Geometry: final body of the model. Coordinates: model frame, mm. A direction names the side the tool comes from. Coordinates: 2 decimals unless noted, no trailing zeros. Write each loop counter-clockwise with the first axis right and the second up, starting at its lowest first coordinate (ties: lowest second). Pieces come first, ordered by that corner, then holes.
from build123d import *

# Parameters (mm, degrees)
EXTRUDE_THIN1_DEPTH = 2
SKETCH2_R           = 3
BOSS_EXTRUDE1_DEPTH = 2
SKETCH3_R           = 1.5
CUT_EXTRUDE1_DEPTH  = 23.73845331
SKETCH4_R           = 1.5
BOSS_EXTRUDE2_DEPTH = 2.1
EXTRUDE_THIN2_DEPTH = 2
EXTRUDE_THIN3_DEPTH = 2
SKETCH7_W           = 1.2
SKETCH7_H           = 23.975911633
EXTRUDE_THIN4_DEPTH = 2


with BuildPart() as part:
    # Sketch1 → Extrude-Thin1 (new body)
    with BuildSketch(Plane(origin=(0, 0, 0), x_dir=(1, 0, 0), z_dir=(0, 1, 0))):
        Polygon((-2.187026997, 14.752740827), (-17.187026997, -11.228021286), (12.812973003, -11.228021286), align=None)
        Polygon((-2.187026997, 12.352740827), (-15.108566028, -10.028021286), (10.734512034, -10.028021286), align=None, mode=Mode.SUBTRACT)
    extrude(amount=EXTRUDE_THIN1_DEPTH)

    # Sketch2 → Boss-Extrude1 (add)
    with BuildSketch(Plane(origin=(0, 0, 0), x_dir=(1, 0, 0), z_dir=(0, 1, 0))):
        with Locations((-9.687026997, 1.76235977)):
            Circle(SKETCH2_R)
        with Locations((5.312973003, 1.76235977)):
            Circle(SKETCH2_R)
        with Locations((-2.187026997, -11.228021286)):
            Circle(SKETCH2_R)
    extrude(amount=BOSS_EXTRUDE1_DEPTH)

    # Sketch3 → Cut-Extrude1 (cut, through all)
    with BuildSketch(Plane(origin=(0, 0, 0), x_dir=(1, 0, 0), z_dir=(0, 1, 0))):
        with Locations(Location((-9.687026997, 1.76235977, 0), (0, 0, 270))):
            Circle(SKETCH3_R)
        with Locations(Location((5.312973003, 1.76235977, 0), (0, 0, 270))):
            Circle(SKETCH3_R)
    extrude(amount=CUT_EXTRUDE1_DEPTH, mode=Mode.SUBTRACT)

    # Sketch4 → Boss-Extrude2 (add)
    with BuildSketch(Plane(origin=(0, 2, 0), x_dir=(1, 0, 0), z_dir=(0, 1, 0))):
        with Locations(Location((-2.187026997, -11.228021286, 0), (0, 0, 270))):
            Circle(SKETCH4_R)
    extrude(amount=BOSS_EXTRUDE2_DEPTH)

    # Sketch5 → Extrude-Thin2 (add)
    with BuildSketch(Plane(origin=(0, 0, 0), x_dir=(1, 0, 0), z_dir=(0, 1, 0))):
        Polygon((-5.388180626, 8.61177443), (2.926064281, 1.202897678), (-10.696610006, -3.999977956), (-6.443313294, -10.266536854), (-7.436211418, -10.940445836), (-12.540725216, -3.419753411), (0.654437519, 1.619843752), (-6.186526415, 7.715870417), align=None)
    extrude_thin2 = extrude(amount=EXTRUDE_THIN2_DEPTH)

    # Sketch6 → Extrude-Thin3 (add)
    with BuildSketch(Plane(origin=(0, 0, 0), x_dir=(1, 0, 0), z_dir=(0, 1, 0))):
        Polygon((-15.108566028, -10.028021286), (6.483160233, -1.838837543), (6.05761065, -0.716827048), (-15.534115611, -8.906010791), align=None)
    extrude_thin3 = extrude(amount=EXTRUDE_THIN3_DEPTH)

    # Mirror1: Extrude-Thin2, Extrude-Thin3 across plane
    add(extrude_thin2.mirror(Plane(origin=(-2.187026997, 0, 0), x_dir=(0, 0, 1), z_dir=(1, 0, 0))))
    add(extrude_thin3.mirror(Plane(origin=(-2.187026997, 0, 0), x_dir=(0, 0, 1), z_dir=(1, 0, 0))))

    # Sketch7 → Extrude-Thin4 (add)
    with BuildSketch(Plane(origin=(0, 0, 0), x_dir=(1, 0, 0), z_dir=(0, 1, 0))):
        with Locations((-2.187026997, 0.75993453)):
            Rectangle(SKETCH7_W, SKETCH7_H)
    extrude(amount=EXTRUDE_THIN4_DEPTH)


solid = part.part
Item 1: Set-up query: faces 1 (the flat face through (7, 1, 11.228)), 2 (the flat face through (-11, 1, 11.228)), 3 (the flat face through (-12, 1, 10.028)). Return all of +Z, -Z, +X, -X, +Y, -Y with unobstructed straight access to the full face (end or side cutting, diameter ignored); none if empty.
Derived:
face 1: +Z, +X, +Y, -Y
face 2: +Z, -X, +Y, -Y
face 3: +Y, -Y
Item 2: Section C-C, the plane z = 5. Output: boundary loops of the cut face in (x, y).
Derived:
outline: (-13.59, 0) - (-12.21, 0) - (-12.21, 2) - (-13.59, 2) - close; (-11.47, 0) - (-10.02, 0) - (-10.02, 2) - (-11.47, 2) - close; (-5.24, 0) - (0.86, 0) - (0.86, 2) - (-5.24, 2) - close; (5.64, 0) - (7.09, 0) - (7.09, 2) - (5.64, 2) - close; (7.83, 0) - (9.22, 0) - (9.22, 2) - (7.83, 2) - close
Item 3: Pin query (flat end, axial travel): pin 1 (1.6 mm diameter, centred on y = 1.5, z = 3, fed in from -X); pin 2 (2 mm diameter, centred on x = -10, y = 0.5, fed in from -Z); pin 3 (0.6 mm diameter, centred on y = 1.5, z = 6.5, fed in from +X); pin 4 (1.8 mm diameter, centred on x = -9.69, z = -1.76, fed in from -Y). Return the tip coordinate at first contact, or that it passes through.
Derived:
pin 1: stops at x = -12.9
pin 2: stops at z = -4.76
pin 3: stops at x = 10.26
pin 4: passes through
Item 4: Section B-B, the plane z = 11.75. Output: boundary loops of the cut face in (x, y).
Derived:
outline: (-5.14, 0) - (0.77, 0) - (0.77, 2) - (-0.78, 2) - (-0.78, 4.1) - (-3.59, 4.1) - (-3.59, 2) - (-5.14, 2) - close
Item 5: Material intervals for probe 1 along Z at (x, y) = (-14, 1.05); probe 2 along Z at (x, y) = (9.5, 1.35); probe 3 along Z at (x, y) = (-6, 1.15), sorted ascending.
Derived:
probe 1: z = 5.71 to 8.11, 8.32 to 9.61, 10.03 to 11.23
probe 2: z = 5.49 to 7.89, 8.28 to 9.56, 10.03 to 11.23
probe 3: z = -8.15 to -5.75, -2.36 to -0.71, 0.92 to 2.21, 2.4 to 3.68, 5.29 to 6.57, 10.03 to 11.23
Item 6: Section D-D, the plane y = 2.4. Output: boundary loops of the cut face in (x, z), plus the area to 3 significant figures.
Derived:
outline: circle Ø3 at (-2.19, 11.23)
area: 7.07 mm2
Item 7: Section A-A, the plane z = -8.5. Output: boundary loops of the cut face in (x, y), plus the area to 3 significant figures.
Derived:
outline: (-5.8, 0) - (-4.41, 0) - (-4.41, 2) - (-5.8, 2) - close; (-2.79, 0) - (-1.59, 0) - (-1.59, 2) - (-2.79, 2) - close; (0.04, 0) - (1.42, 0) - (1.42, 2) - (0.04, 2) - close
area: 7.94 mm2
